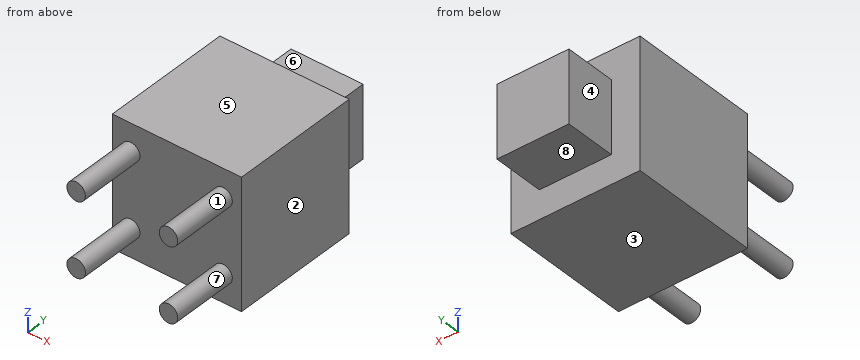
from build123d import *

# Parameters (mm, degrees)
SKETCH_1_W      = 7
SKETCH_1_H      = 7
EXTRUDE_1_DEPTH = 7.1
SKETCH_2_W      = 3.9
SKETCH_2_H      = 3.9
EXTRUDE_2_DEPTH = 2.8
SKETCH_3_R      = 0.5
EXTRUDE_3_DEPTH = 3.6


with BuildPart() as part:
    # 草图1 → 凸台-拉伸1 (new body)
    with BuildSketch(Plane(origin=(0, 0, 0), x_dir=(1, 0, 0), z_dir=(0, 1, 0))):
        with Locations((3.5, 3.5)):
            Rectangle(SKETCH_1_W, SKETCH_1_H)
    extrude(amount=EXTRUDE_1_DEPTH)

    # 草图2 → 凸台-拉伸2 (add)
    with BuildSketch(Plane(origin=(0, 7.1, 0), x_dir=(1, 0, 0), z_dir=(0, 1, 0))):
        with Locations((3.5, 3.5)):
            Rectangle(SKETCH_2_W, SKETCH_2_H)
    extrude(amount=EXTRUDE_2_DEPTH)

    # 草图3 → 凸台-拉伸3 (add)
    with BuildSketch(Plane.XZ):
        with Locations(Location((1, -1.5, 0), (0, 0, 270))):
            Circle(SKETCH_3_R)
        with Locations(Location((6, -1.5, 0), (0, 0, 270))):
            Circle(SKETCH_3_R)
        with Locations(Location((6, -5.5, 0), (0, 0, 270))):
            Circle(SKETCH_3_R)
        with Locations(Location((1, -5.5, 0), (0, 0, 270))):
            Circle(SKETCH_3_R)
    extrude(amount=EXTRUDE_3_DEPTH)


solid = part.part
Design review of the part built by this model. Coordinates are the model's own, in mm. Face numbers are marked on the shaded views. A direction names the side the tool comes from. Round coordinates to 2 decimals unless told otherwise and drop trailing zeros. Order: outer loops, then holes, each group sorted by start corner. A loop starts at its lowest first (then second) coordinate and runs counter-clockwise, first axis right, second up.
1) For L1, parallel to Y at x = 3, z = -2.75; L2, parallel to Y at x = 6.5, z = -5.25; L3, parallel to X at y = 7.75, z = -5, list the stretches that pass through material, from the lowest coordinate up.
The answers:
L1: y = 0 to 9.9
L2: y = 0 to 7.1
L3: x = 1.55 to 5.45
2) Consider section C-C (y = 7.75). State the section outline as (x, z) points, plus the area to 3 significant figures.
The answers:
outline: (1.55, -5.45) - (5.45, -5.45) - (5.45, -1.55) - (1.55, -1.55) - close
area: 15.2 mm2
3) Consider section B-B (z = -4.75). State the section outline as (x, y) points, plus the area to 3 significant figures.
The answers:
outline: (0, 0) - (7, 0) - (7, 7.1) - (5.45, 7.1) - (5.45, 9.9) - (1.55, 9.9) - (1.55, 7.1) - (0, 7.1) - close
area: 60.6 mm2
4) Consider section A-A (x = 1). State the section outline as (y, z) points, plus the area to 3 significant figures.
The answers:
outline: (-3.6, -6) - (0, -6) - (0, -7) - (7.1, -7) - (7.1, 0) - (0, 0) - (0, -1) - (-3.6, -1) - (-3.6, -2) - (0, -2) - (0, -5) - (-3.6, -5) - close
area: 56.9 mm2
5) Draft analysis for pull direction X (two halves, no side actions). For the marked faces 1, 2, 3 and 4, state which applies: released by +X, released by -X, zero draft, split by the parting line, or undercut.
The answers:
face 1: undercut
face 2: released by +X
face 3: zero draft
face 4: released by -X
6) Machinability: for the marked faces 5, 6, 7 and 8, which of the approach directions +Z, -Z, +X, -X, +Y, -Y give a long, thin tool a straight path to every point of the face, cutting with its end or side? Answer none if there is none.
The answers:
face 5: +Z, +X, -X, +Y, -Y
face 6: +Z, +X, -X, +Y
face 7: -Y
face 8: -Z, +X, -X, +Y
7) Consider section D-D (x = 5.75). State the section outline as (y, z) points, plus the area to 3 significant figures.
The answers:
outline: (-3.6, -5.93) - (0, -5.93) - (0, -7) - (7.1, -7) - (7.1, 0) - (0, 0) - (0, -1.07) - (-3.6, -1.07) - (-3.6, -1.93) - (0, -1.93) - (0, -5.07) - (-3.6, -5.07) - close
area: 55.9 mm2
8) Clearance check with flat-ended pins moving along their axes: pin 1 Ø0.8 at (y, z) = (8.5, -3) entering from -X; pin 2 Ø3 at (x, y) = (3, 9) entering from -Z. State where each tip first meets the part, or that it passes through.
The answers:
pin 1: stops at x = 1.55
pin 2: stops at z = -5.45
